```python
from build123d import *

# Parameters (mm, degrees)
SKETCH1_W           = 10
SKETCH1_H           = 10
BOSS_EXTRUDE1_DEPTH = 8.89
SKETCH2_R           = 2.5
CUT_EXTRUDE1_DEPTH  = 11.43
FILLET1_R           = 1.397


with BuildPart() as part:
    # Sketch1 → Boss-Extrude1 (new, symmetric)
    with BuildSketch(Plane(origin=(0, 0, 0), x_dir=(1, 0, 0), z_dir=(0, 1, 0))):
        Rectangle(SKETCH1_W, SKETCH1_H)
    extrude(amount=BOSS_EXTRUDE1_DEPTH, both=True)

    # Sketch2 → Cut-Extrude1 (cut)
    with BuildSketch(Plane.XZ.offset(8.89)):
        with Locations(Location((0, 0, 0), (0, 0, 270))):
            Circle(SKETCH2_R)
    extrude(amount=-CUT_EXTRUDE1_DEPTH, mode=Mode.SUBTRACT)

    # Fillet1
    fillet1_edges = [part.edges().sort_by_distance(p)[0] for p in [
        (5, 0, -5),
        (5, 0, 5),
        (-5, 0, 5),
        (-5, 0, -5),
    ]]
    fillet(fillet1_edges, radius=FILLET1_R)


solid = part.part
```
Geometry: final body of the model. Coordinates: model frame, mm. A direction names the side the tool comes from. Give positions to 0.01 mm unless a question says otherwise; leave off trailing zeros. Order: outer loops, then holes, each group sorted by start corner. A loop starts at its lowest first (then second) coordinate and runs counter-clockwise, first axis right, second up. Notation, with made-up numbers: (-16, 89) -> (21, 89) arc R17 cw to (21, 112) -> close; hole circle Ø9 at (-24.5, 6). An arc over 180 degrees is marked (long way). Write each question's results on one line, items separated by ' | '. Start each with the question number.
1) Section C-C (x = 0). Return loops of the section in (y, z), then the cut area to 3 significant figures.
2) Section A-A (y = 1.25). Return loops of the section in (x, z).
3) Line query: line 1 (X direction, y = -6.25, z = 0); line 2 (Y direction, x = -0.75, z = -2); line 3 (Z direction, x = -1.25, y = -4.75). Output: solid intervals per line, ascending. Write a range as from..to.
4) Set-up query: faces 1 (the flat face through (0, 2.54, 0)), 2 (the cylindrical face through (4.58, 0.12, 4.6)). Return all of +Z, -Z, +X, -X, +Y, -Y with unobstructed straight access to the full face (end or side cutting, diameter ignored); none if empty.
5) First-contact query: pin 1 (4.5 mm diameter, centred on x = 0, z = 0, fed in from -Y). Flat tip, straight axial feed; report the tip coordinate or a pass-through.
6) Section B-B (z = -1.5). Return loops of the section in (x, y), then the cut area to 3 significant figures.
Calculated:
1) outline: (-8.89, -5) -> (8.89, -5) -> (8.89, 5) -> (-8.89, 5) -> (-8.89, 2.5) -> (2.54, 2.5) -> (2.54, -2.5) -> (-8.89, -2.5) -> close | area: 121 mm2
2) outline: (-5, -3.6) arc R1.4 ccw to (-3.6, -5) -> (3.6, -5) arc R1.4 ccw to (5, -3.6) -> (5, 3.6) arc R1.4 ccw to (3.6, 5) -> (-3.6, 5) arc R1.4 ccw to (-5, 3.6) -> close; hole circle Ø5 at (0, 0)
3) line 1: -5..-2.5, 2.5..5 | line 2: 2.54..8.89 | line 3: -5..-2.17, 2.17..5
4) face 1: -Y | face 2: +Z, +X, +Y, -Y
5) pin 1: y = 2.54
6) outline: (-5, -8.89) -> (-2, -8.89) -> (-2, 2.54) -> (2, 2.54) -> (2, -8.89) -> (5, -8.89) -> (5, 8.89) -> (-5, 8.89) -> close | area: 132 mm2
